```python
from build123d import *

# Parameters (mm, degrees)
CHAMFER1_SIZE = 0.5


with BuildPart() as part:
    # Sketch2 → Revolve1 (revolve)
    with BuildSketch(Plane(origin=(0, 0, 0), x_dir=(0, 0, -1), z_dir=(1, 0, 0)), mode=Mode.PRIVATE) as revolve1_sk:
        Polygon((15, 8.9), (11, 8.9), (11, 11.1), (7, 11.1), (7, 14.15), (0, 14.15), (0, 7.1), (5, 7.1), (8.637306696, 5), (15, 5), align=None)
    revolve(revolve1_sk.sketch.rotate(Axis((0, 0, 0), (0, 0, -1)), 90), axis=Axis((0, 0, 0), (0, 0, -1)))

    # Chamfer1
    chamfer1_edges = [part.edges().sort_by_distance(p)[0] for p in [
        (-14.15, 0, -7),
        (-11.1, 0, -11),
        (-8.9, 0, -15),
        (-7.1, 0, 0),
        (-14.15, 0, 0),
    ]]
    chamfer(chamfer1_edges, length=CHAMFER1_SIZE)


solid = part.part
```
Check sheet for the modelled part. Datum: model origin and axes. Units: mm. A direction names the side the tool comes from. Round coordinates to 2 decimals unless told otherwise and drop trailing zeros. Order: outer loops, then holes, each group sorted by start corner. A loop starts at its lowest first (then second) coordinate and runs counter-clockwise, first axis right, second up. Notation, with made-up numbers: (74.25, 73.5) -> (106.25, 73.5) arc R17 ccw to (106.25, 90.5) -> close; hole circle Ø11 at (-22, 8). An arc over 180 degrees is marked (long way). One line per item, written item: value. Start each with the question number.
Q1. Mould release check, pull along X, two halves, no side actions. Record for faces 4 (the face through (-2, 11.1, -7)), 5 (the face through (2.35, 4.53, -8.46)), 6 (the face through (-1.445, -11.006, -8.726)): pulls with the +X half, pulls with the -X half, needs draft (parallel to the pull), parting line crosses it, or undercut.
Q2. Gauge pin test, flat ends, axial feed: pin 1 Ø4 at (y, z) = (3.5, -3.5) entering from -X; pin 2 Ø8 at (y, z) = (-7.5, -5.5) entering from -X; pin 3 Ø5 at (y, z) = (5.5, -12.5) entering from -X. Record the tip position at first contact, or that the pin passes through.
Q3. Cross-section at C-C (z = -12.75). Record the boundary of the cut face in (x, y), and give its area (3 significant figures).
Q4. Set-up check for faces 1 (the face through (2, -9, -11)), 2 (the face through (6, 6, 0)), 3 (the face through (-0.92, -7.04, -2.78)): record each of +Z, -Z, +X, -X, +Y, -Y from which the full face is reachable in a straight line by a thin tool's end or side.
Q5. Thickness scan on line 1 (Y direction, x = 0, z = -4); line 2 (Z direction, x = -11.5, y = -7); line 3 (Y direction, x = 0, z = -12). Record the ranges inside material, lowest first.
Completed:
1. face 4: needs draft
1. face 5: undercut
1. face 6: parting line crosses it
2. pin 1: stops at x = -14.07
2. pin 2: stops at x = -13.71
2. pin 3: stops at x = -10.35
3. outline: circle Ø17.8 at (0, 0); hole circle Ø10 at (0, 0)
3. area: 170 mm²
4. face 1: -Z
4. face 2: +Z, +X, -X, +Y, -Y
4. face 3: +Z
5. line 1: y = -14.15 to -7.1, 7.1 to 14.15
5. line 2: z = -7 to 0
5. line 3: y = -8.9 to -5, 5 to 8.9
